```python
from build123d import *

# Parameters (mm, degrees)
SKETCH1_R           = 14.2875
BOSS_EXTRUDE1_DEPTH = 3.175
FILLET2_R           = 6.35


with BuildPart() as part:
    # Sketch1 → Boss-Extrude1 (new body)
    with BuildSketch(Plane(origin=(0, 0, 0), x_dir=(1, 0, 0), z_dir=(0, 1, 0))):
        with BuildLine():
            Line((71.172208723, -15.271936024), (109.397864591, 35.52897381))
            ThreePointArc((109.397864591, 35.52897381), (104.373791891, 71.096918557), (68.805847145, 66.072845858))
            Line((68.805847145, 66.072845858), (38.201154945, 25.4))
            Line((38.201154945, 25.4), (0, 25.4))
            ThreePointArc((0, 25.4), (-25.4, 0), (0, -25.4))
            Line((0, -25.4), (50.8762, -25.4))
            ThreePointArc((50.8762, -25.4), (62.217558494, -22.727375288), (71.172208723, -15.271936024))
        make_face()
        with Locations(Location((89.101855868, 50.800909834, 0), (0, 0, 270))):
            Circle(SKETCH1_R, mode=Mode.SUBTRACT)
        with Locations(Location((50.8762, 0, 0), (0, 0, 270))):
            Circle(SKETCH1_R, mode=Mode.SUBTRACT)
        with Locations(Location((0, 0, 0), (0, 0, 270))):
            Circle(SKETCH1_R, mode=Mode.SUBTRACT)
    extrude(amount=BOSS_EXTRUDE1_DEPTH)

    # Fillet2
    fillet2_edges = [part.edges().sort_by_distance(p)[0] for p in [
        (38.201154945, 1.5875, -25.4),
    ]]
    fillet(fillet2_edges, radius=FILLET2_R)


solid = part.part
```
Source: CAD feature listing. Evaluate the final solid. Frame: model axes, mm. A direction names the side the tool comes from. Round coordinates to 2 decimals unless told otherwise and drop trailing zeros. Loops run counter-clockwise (first coordinate to the right, second up) from the corner with the lowest first, then second, coordinate; pieces in that order, holes last. Notation, with made-up numbers: M 28,46.5 L 62,46.5 A14 ccw 62,65.5 Z; hole C -16,-32 d8. An arc over 180 degrees is marked long. Use a Markdown table: item, result. Add a question column.
1. Contact query for flat-ended pins moving along their axis: pin 1 (5 mm diameter, centred on x = 8, z = 11, fed in from +Y) (3 decimals); pin 2 (1 mm diameter, centred on y = 1, z = -56, fed in from -X). Output: stop coordinate, or through.
2. Cut plane D-D, the plane y = 0.6. State how many separate pieces and enclosed holes the cut face has, and give its area (3 significant figures).
3. Cut plane A-A, the plane x = 93.5. Output: boundary loops of the cut face in (y, z) (3 decimals), and give its area (3 significant figures).
4. Cut plane B-B, the plane z = -50.5. Output: boundary loops of the cut face in (x, y) (3 decimals).
5. Cut plane C-C, the plane z = 0. Output: boundary loops of the cut face in (x, y) (1 decimal), and give its area (3 significant figures).
6. Set-up query: faces 1 (the flat face through (18, 2, -25.4)), 2 (the cylindrical face through (104.816, 1.565, -70.756)). Return all of +Z, -Z, +X, -X, +Y, -Y with unobstructed straight access to the full face (end or side cutting, diameter ignored); none if empty.
7. Pull-direction query (X, two-part tool) for faces 3 (the cylindrical face through (0.628, 1.565, -14.274)), 4 (the cylindrical face through (37.904, 1.61, -26.087)), 5 (the flat face through (44, 0, -15)); classes: +X half, -X half, draft (parallel to the pull), parting line (faces both ways), or undercut.
8. Ray query, line 1 along X through (y, z) = (0.75, 0); line 2 along X through (y, z) = (2.45, -13); line 3 along X through (y, z) = (0.2, -41). Return the intervals inside material, ascending. Write a range as [from, to].
Solution:
| question | item | result |
|---|---|---|
| 1 | pin 1 | stops at y = 3.175 |
| 1 | pin 2 | stops at x = 60.85 |
| 2 | separate pieces | 1 |
| 2 | enclosed holes | 3 |
| 2 | area | 5,900 mm2 |
| 3 | outline | M 0,-75.817 L 3.175,-75.817 L 3.175,-64.395 L 0,-64.395 Z; M 0,-37.207 L 3.175,-37.207 L 3.175,-14.401 L 0,-14.401 Z |
| 3 | area | 109 mm2 |
| 4 | outline | M 57.088,0 L 74.818,0 L 74.818,3.175 L 57.088,3.175 Z; M 103.386,0 L 114.5,0 L 114.5,3.175 L 103.386,3.175 Z |
| 5 | outline | M -25.4,0 L -14.3,0 L -14.3,3.2 L -25.4,3.2 Z; M 14.3,0 L 36.6,0 L 36.6,3.2 L 14.3,3.2 Z; M 65.2,0 L 82.7,0 L 82.7,3.2 L 65.2,3.2 Z |
| 5 | area | 162 mm2 |
| 6 | face 1 | -Z, -X, +Y, -Y |
| 6 | face 2 | +Y, -Y |
| 7 | face 3 | undercut |
| 7 | face 4 | -X half |
| 7 | face 5 | draft |
| 8 | line 1 | x = [-25.4, -14.29], [14.29, 36.59], [65.16, 82.66] |
| 8 | line 2 | x = [-21.82, -5.93], [5.93, 44.95], [56.8, 92.45] |
| 8 | line 3 | x = [49.94, 78.71], [99.5, 112.53] |
